Build history of the part. All positions in model axes, mm. A direction names the side the tool comes from. Round coordinates to 2 decimals unless told otherwise and drop trailing zeros. Loops run counter-clockwise (first coordinate to the right, second up) from the corner with the lowest first, then second, coordinate; pieces in that order, holes last. Notation, with made-up numbers: (-21.75, -28.75) - (36.25, -28.75) arc R20 ccw to (36.25, -16.75) - close; hole circle Ø2 at (24.5, 34.25). An arc over 180 degrees is marked (long way). Use one line per item in the form item = value. Start each with the question number.
Q1. Mould opens along X. For faces 1 (the face through (-3.8, -8, -42.5)), 2 (the face through (-10.44, 1.94, -34.93)), 3 (the face through (-15.6, 0.6, -37.1)), 4 (the face through (-1.3, -5, -43)) say: released by +X, released by -X, zero draft, split by the parting line, or undercut.
Q2. Saw through at C-C (z = -36.3). Give the cut face in (x, y).
Q3. Saw through at D-D (x = 15). Give the cut face in (y, z), then the cut area to 3 significant figures.
Q4. Pin check, flat tips, straight feed: pin 1 (1 mm diameter, centred on y = 0.5, z = -1, fed in from +X); pin 2 (0.6 mm diameter, centred on y = 0.5, z = -2, fed in from -X); pin 3 (11 mm diameter, centred on x = 5, z = -15.5, fed in from -Y). Stop position of each tip, or through.
Q5. 3-axis set-ups, long thin cutter, end or side, ignore diameter. For faces 5 (the face through (0, -1, -32.5)), 6 (the face through (0, -1, -28)), 7 (the face through (-8.9, -5, -43)), 8 (the face through (-8, 1, -2)): which of +Z, -Z, +X, -X, +Y, -Y reach the whole face in a straight line?
Q6. Saw through at A-A (y = -1). Give the cut face in (x, z), then the cut area to 3 significant figures.
Q7. Saw through at B-B (y = -7.25). Give the cut face in (x, z), then the cut area to 3 significant figures.
Q8. Drill centre lines: line 1 (X direction, y = 0.6, z = -6.3); line 2 (Z direction, x = 6.5, y = -1.25); line 3 (Y direction, x = 16, z = -6). Where is each one in solid material? Low to high.
```python
from build123d import *

# Parameters (mm, degrees)
SKETCH_1_R      = 1
EXTRUDE_1_DEPTH = 1.2
SKETCH_2_R      = 17.16
EXTRUDE_2_DEPTH = 1.5
SKETCH_3_W      = 12
SKETCH_3_H      = 4.5
SKETCH_3_W_2    = 22.86
SKETCH_3_H_2    = 2.54
EXTRUDE_3_DEPTH = 2
SKETCH_4_R      = 0.5
EXTRUDE_4_DEPTH = 8


with BuildPart() as part:
    # 草图1 → 凸台-拉伸1 (new body)
    with BuildSketch(Plane(origin=(0, 0, 0), x_dir=(1, 0, 0), z_dir=(0, 1, 0))):
        Polygon((-12, 44), (12, 44), (18, 38), (18, 6), (12, 0), (8, 0), (8, 3), (-8, 3), (-8, 0), (-12, 0), (-18, 6), (-18, 38), align=None)
        with Locations(Location((15, 6.3, 0), (0, 0, 270))):
            Circle(SKETCH_1_R, mode=Mode.SUBTRACT)
        with Locations(Location((15, 36.3, 0), (0, 0, 90))):
            Circle(SKETCH_1_R, mode=Mode.SUBTRACT)
        with Locations(Location((-15, 6.3, 0), (0, 0, 90))):
            Circle(SKETCH_1_R, mode=Mode.SUBTRACT)
        with Locations(Location((-15, 36.3, 0), (0, 0, 270))):
            Circle(SKETCH_1_R, mode=Mode.SUBTRACT)
    extrude(amount=EXTRUDE_1_DEPTH)

    # 草图2 → 凸台-拉伸2 (add)
    with BuildSketch(Plane(origin=(0, 1.2, 0), x_dir=(1, 0, 0), z_dir=(0, 1, 0))):
        with Locations(Location((0, 21.31, 0), (0, 0, 270))):
            Circle(SKETCH_2_R)
    extrude(amount=EXTRUDE_2_DEPTH)

    # 草图3 → 凸台-拉伸3 (add)
    with BuildSketch(Plane.XZ):
        with Locations((0, -30.25)):
            Rectangle(SKETCH_3_W, SKETCH_3_H)
        with Locations((0, -42.73)):
            Rectangle(SKETCH_3_W_2, SKETCH_3_H_2)
    extrude(amount=EXTRUDE_3_DEPTH)

    # 草图4 → 凸台-拉伸4 (add)
    with BuildSketch(Plane.XZ):
        with Locations(Location((-1.27, -42.5, 0), (0, 0, 90))):
            Circle(SKETCH_4_R)
        with Locations(Location((-3.81, -42.5, 0), (0, 0, 90))):
            Circle(SKETCH_4_R)
        with Locations(Location((-6.35, -42.5, 0), (0, 0, 90))):
            Circle(SKETCH_4_R)
        with Locations(Location((-8.89, -42.5, 0), (0, 0, 90))):
            Circle(SKETCH_4_R)
        with Locations(Location((8.89, -42.5, 0), (0, 0, 90))):
            Circle(SKETCH_4_R)
        with Locations(Location((6.35, -42.5, 0), (0, 0, 90))):
            Circle(SKETCH_4_R)
        with Locations(Location((3.81, -42.5, 0), (0, 0, 90))):
            Circle(SKETCH_4_R)
        with Locations(Location((1.27, -42.5, 0), (0, 0, 90))):
            Circle(SKETCH_4_R)
    extrude(amount=EXTRUDE_4_DEPTH)


solid = part.part
```
Report:
q1.face_1 = zero draft
q1.face_2 = split by the parting line
q1.face_3 = undercut
q1.face_4 = undercut
q2.outline = (-18, 0) - (-16, 0) - (-16, 1.2) - (-18, 1.2) - close; (-14, 0) - (14, 0) - (14, 1.2) - (8.35, 1.2) - (8.35, 2.7) - (-8.35, 2.7) - (-8.35, 1.2) - (-14, 1.2) - close; (16, 0) - (18, 0) - (18, 1.2) - (16, 1.2) - close
q3.outline = (0, -41) - (1.2, -41) - (1.2, -37.3) - (0, -37.3) - close; (0, -35.3) - (1.2, -35.3) - (1.2, -29.64) - (2.7, -29.64) - (2.7, -12.98) - (1.2, -12.98) - (1.2, -7.3) - (0, -7.3) - close; (0, -5.3) - (1.2, -5.3) - (1.2, -3) - (0, -3) - close
q3.area = 65.8 mm²
q4.pin_1 = 13.5
q4.pin_2 = -14.3
q4.pin_3 = 0
q5.face_5 = +X, -X, -Y
q5.face_6 = +Z, +X, -X, -Y
q5.face_7 = -Y
q5.face_8 = +Z, +Y, -Y
q6.outline = (-11.43, -44) - (11.43, -44) - (11.43, -41.46) - (-11.43, -41.46) - close; (-6, -32.5) - (6, -32.5) - (6, -28) - (-6, -28) - close
q6.area = 112 mm²
q7.outline = circle Ø1 at (-8.89, -42.5); circle Ø1 at (-6.35, -42.5); circle Ø1 at (-3.81, -42.5); circle Ø1 at (-1.27, -42.5); circle Ø1 at (1.27, -42.5); circle Ø1 at (3.81, -42.5); circle Ø1 at (6.35, -42.5); circle Ø1 at (8.89, -42.5)
q7.area = 6.28 mm²
q8.line_1 = -18 to -16, -14 to 14, 16 to 18
q8.line_2 = -44 to -41.46
q8.line_3 = 0 to 1.2
